```python
from build123d import *

# Parameters (mm, degrees)
SKETCH1_W                      = 36
SKETCH1_H                      = 36
EXTRUDE_THIN1_DEPTH            = 730
CUT_EXTRUDE1_REACH             = 734.189
SKETCH2_R                      = 4
CUT_EXTRUDE1_DIRECTION_2_DEPTH = 733.188500319
CUT_EXTRUDE4_REACH             = 734.189
SKETCH5_R                      = 2.5
CUT_EXTRUDE6_REACH             = 734.189
SKETCH6_R                      = 4


with BuildPart() as part:
    # Sketch1 → Extrude-Thin1 (new body)
    with BuildSketch(Plane(origin=(0, 0, 0), x_dir=(1, 0, 0), z_dir=(0, 1, 0))):
        with BuildLine():
            Line((2, 0), (38, 0))
            ThreePointArc((38, 0), (39.414213562, -0.585786438), (40, -2))
            Line((40, -2), (40, -38))
            ThreePointArc((40, -38), (39.414213562, -39.414213562), (38, -40))
            Line((38, -40), (2, -40))
            ThreePointArc((2, -40), (0.585786438, -39.414213562), (0, -38))
            Line((0, -38), (0, -2))
            ThreePointArc((0, -2), (0.585786438, -0.585786438), (2, 0))
        make_face()
        with Locations((20, -20)):
            Rectangle(SKETCH1_W, SKETCH1_H, mode=Mode.SUBTRACT)
    extrude(amount=EXTRUDE_THIN1_DEPTH)

    # Cut-Extrude1: up to this face of the body (flat: up to its plane)
    cut_extrude1_end = Plane(part.part.faces().sort_by_distance((20, 365, 0))[0])
    # Sketch2 → Cut-Extrude1 (cut, up to the picked face)
    with BuildSketch(Plane.XY.offset(40), mode=Mode.PRIVATE) as cut_extrude1_sk1:
        with Locations((20, 15)):
            Circle(SKETCH2_R)
    cut_extrude1_tool1 = split(extrude(cut_extrude1_sk1.sketch, amount=-CUT_EXTRUDE1_REACH, mode=Mode.PRIVATE), bisect_by=cut_extrude1_end, keep=Keep.BOTH, mode=Mode.PRIVATE)
    add(cut_extrude1_tool1.solids().sort_by(Axis((20, 15, 40), (0, 0, -1)))[0], mode=Mode.SUBTRACT)

    # Sketch2 → Cut-Extrude1 direction 2 (cut)
    with BuildSketch(Plane.XY.offset(40)):
        with Locations((20, 15)):
            Circle(SKETCH2_R)
    extrude(amount=CUT_EXTRUDE1_DIRECTION_2_DEPTH, mode=Mode.SUBTRACT)

    # Cut-Extrude4: up to this face of the body (flat: up to its plane)
    cut_extrude4_end = Plane(part.part.faces().sort_by_distance((40, 365, 20))[0])
    # Sketch5 → Cut-Extrude4 (cut, up to the picked face)
    with BuildSketch(Plane.ZY, mode=Mode.PRIVATE) as cut_extrude4_sk1:
        with Locations((20, 715)):
            Circle(SKETCH5_R)
    cut_extrude4_tool1 = split(extrude(cut_extrude4_sk1.sketch, amount=-CUT_EXTRUDE4_REACH, mode=Mode.PRIVATE), bisect_by=cut_extrude4_end, keep=Keep.BOTH, mode=Mode.PRIVATE)
    add(cut_extrude4_tool1.solids().sort_by(Axis((0, 715, 20), (1, 0, 0)))[0], mode=Mode.SUBTRACT)

    # Cut-Extrude6: up to this face of the body (flat: up to its plane)
    cut_extrude6_end = Plane(part.part.faces().sort_by_distance((0, 364.738303945, 20))[0])
    # Sketch6 → Cut-Extrude6 (cut, up to the picked face)
    with BuildSketch(Plane(origin=(40, 0, 0), x_dir=(0, 0, -1), z_dir=(1, 0, 0)), mode=Mode.PRIVATE) as cut_extrude6_sk1:
        with Locations((-20, 690)):
            Circle(SKETCH6_R)
    cut_extrude6_tool1 = split(extrude(cut_extrude6_sk1.sketch, amount=-CUT_EXTRUDE6_REACH, mode=Mode.PRIVATE), bisect_by=cut_extrude6_end, keep=Keep.BOTH, mode=Mode.PRIVATE)
    # Sketch6 → Cut-Extrude6 (cut, up to the picked face)
    with BuildSketch(Plane(origin=(40, 0, 0), x_dir=(0, 0, -1), z_dir=(1, 0, 0)), mode=Mode.PRIVATE) as cut_extrude6_sk2:
        with Locations((-20, 614)):
            Circle(SKETCH6_R)
    cut_extrude6_tool2 = split(extrude(cut_extrude6_sk2.sketch, amount=-CUT_EXTRUDE6_REACH, mode=Mode.PRIVATE), bisect_by=cut_extrude6_end, keep=Keep.BOTH, mode=Mode.PRIVATE)
    add(cut_extrude6_tool1.solids().sort_by(Axis((40, 690, 20), (-1, 0, 0)))[0], mode=Mode.SUBTRACT)
    add(cut_extrude6_tool2.solids().sort_by(Axis((40, 614, 20), (-1, 0, 0)))[0], mode=Mode.SUBTRACT)


solid = part.part
```
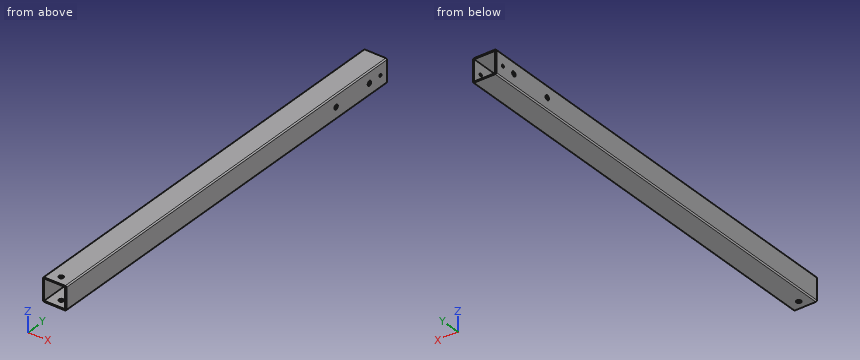
Design review of the part built by this model. Coordinates are the model's own, in mm. Coordinates: 2 decimals unless noted, no trailing zeros. Write each loop counter-clockwise with the first axis right and the second up, starting at its lowest first coordinate (ties: lowest second). Pieces come first, ordered by that corner, then holes.
1) Add section B-B (x = 30.5). Write out the cut boundary in (y, z), plus the area to 3 significant figures.
2) To check wall thickness, follow L1, parallel to Y at x = 0.85, z = 20; L2, parallel to Z at x = 35, y = 77. State the ranges of each line that lie inside material, in increasing order.
3) Add section C-C (y = 438.5). Write out the cut boundary in (x, z).
4) Add section A-A (z = 9.5). Write out the cut boundary in (x, y).
Check result:
1. outline: (0, 0) - (730, 0) - (730, 2) - (0, 2) - close; (0, 38) - (730, 38) - (730, 40) - (0, 40) - close
1. area: 2,920 mm2
2. L1: y = 0 to 610, 618 to 686, 694 to 712.5, 717.5 to 730
2. L2: z = 0 to 2, 38 to 40
3. outline: (0, 2) arc R2 ccw to (2, 0) - (38, 0) arc R2 ccw to (40, 2) - (40, 38) arc R2 ccw to (38, 40) - (2, 40) arc R2 ccw to (0, 38) - close; hole (2, 2) - (38, 2) - (38, 38) - (2, 38) - close
4. outline: (0, 0) - (2, 0) - (2, 730) - (0, 730) - close; (38, 0) - (40, 0) - (40, 730) - (38, 730) - close
